Check sheet for the modelled part. Datum: model origin and axes. Units: mm. A direction names the side the tool comes from. Round coordinates to 2 decimals unless told otherwise and drop trailing zeros. Order: outer loops, then holes, each group sorted by start corner. A loop starts at its lowest first (then second) coordinate and runs counter-clockwise, first axis right, second up. Notation, with made-up numbers: (-28, 87.25) -> (7, 87.25) arc R14 ccw to (7, 105.25) -> close; hole circle Ø3 at (81.5, -22.75). An arc over 180 degrees is marked (long way). Use CSV: the item, a comma, the result in double quotes.
```python
from build123d import *

# Parameters (mm, degrees)
F4_R = 5.99999


# Not quite as in the source:
# - a fillet or chamfer is up to 0.001 mm smaller than in the source, because OpenCascade refuses the exact size


with BuildPart() as f1:
    # F0 (on Front) → F1 (revolve)
    with BuildSketch(Plane.XZ):
        with BuildLine():
            Line((0, 31), (0, 0))
            Line((0, 0), (88, 0))
            Line((88, 0), (88, 16))
            Line((88, 16), (85, 16))
            Line((85, 16), (85, 20))
            Line((85, 20), (68, 20))
            Line((68, 20), (68, 31))
            Line((68, 31), (56, 31))
            ThreePointArc((56, 31), (50, 25), (44, 31))
            Line((44, 31), (0, 31))
        make_face()
    revolve(axis=Axis((55.6183233857, 0, 0), (1, 0, 0)))

    # F2 (on Front) → F3 (revolve, cut)
    with BuildSketch(Plane.XZ):
        Polygon((0, 25), (0, 0), (88, 0), (88, 6), (30, 6), (30, 16), (22, 16), (22, 20.5), (15, 20.5), (15, 12.5), (12, 12.5), (12, 16), (1.5, 16), (1.5, 25), align=None)
    revolve(axis=Axis((-12.6493745584, 0, 0), (-1, 0, 0)), mode=Mode.SUBTRACT)

    # F4 (radius 6 in the source; OpenCascade refuses exactly that, so slightly less here)
    f4_edges = [f1.edges().sort_by_distance(p)[0] for p in [
        (0, 0, -31),
    ]]
    fillet(f4_edges, radius=F4_R)


solid = f1.part
```
Q1. Sectioned sample at B-B, the plane x = 36.5. Enter the section's corners in (y, z).
Result sheet:
outline,"circle Ø62 at (0, 0); hole circle Ø12 at (0, 0)"
Q2. Go/stop test with flat-tipped pins: pin 1 (4 mm diameter, centred on x = 24.5, z = 6.5, fed in from +Y); pin 2 (15 mm diameter, centred on y = 6, z = 10.5, fed in from -X); pin 3 (4 mm diameter, centred on x = 10.5, y = -6.5, fed in from -Z). Record where each tip stops, or that it passes through.
Result sheet:
pin 1,"stops at y = 30.67"
pin 2,"stops at x = 1.5"
pin 3,"stops at z = -30.67"
Q3. Access from +Z, -Z, +X, -X, +Y, -Y to the whole of each face (thin tool, end or side, straight path). Record for faces 1 (the face through (85, -13.43, 8.98)), 2 (the face through (6.68, -15.62, -3.47)), 3 (the face through (22, -11, -12)).
Result sheet:
face 1,"+X"
face 2,"-X"
face 3,"none"
Q4. Scan lines: L1, parallel to Y at x = 32, z = 0; L2, parallel to Y at x = 26.25, z = 0; L3, parallel to X at y = 25, z = 14.5. Record each from-to range of solid material in increasing order.
Result sheet:
L1,"y = -31 to -6, 6 to 31"
L2,"y = -31 to -16, 16 to 31"
L3,"x = 1.44 to 44.38, 55.62 to 68"
Q5. Mould release check, pull along X, two halves, no side actions. Record for faces 4 (the face through (0.74, 7.509, 23.846)), 5 (the face through (25.94, -15.62, -3.47)), 6 (the face through (68, 20.2, 0.4)): pulls with the +X half, pulls with the -X half, needs draft (parallel to the pull), parting line crosses it, or undercut.
Result sheet:
face 4,"needs draft"
face 5,"undercut"
face 6,"pulls with the +X half"
Q6. Sectioned sample at A-A, the plane x = 82. Enter the section's corners in (y, z), then the cut area to 3 significant figures.
Result sheet:
outline,"circle Ø40 at (0, 0); hole circle Ø12 at (0, 0)"
area,"1,140 mm^2"
